Autodesk Inventor part; units mm, degrees
ref_plane "YZ Plane" through (0, 0, 0) normal (1, 0, 0) x (0, 1, 0)
ref_plane "XZ Plane" through (0, 0, 0) normal (0, 1, 0) x (-1, 0, 0)
ref_plane "XY Plane" through (0, 0, 0) normal (0, 0, 1) x (1, 0, 0)
sketch "Sketch1" plane through (0, 0, 0) normal (0, 1, 0) x (-1, 0, 0)
  line L0 (0, 0) -> (88.9, 0)
  line L1 (88.9, 0) -> (76.2, 0) construction
  line L2 (76.2, 0) -> (76.2, -12.7) construction
  line L3 (76.2, -12.7) -> (88.9, -12.7) construction
  line L4 (88.9, -12.7) -> (88.9, 0) construction
  line L5 (0, -349.25) -> (88.9, -349.25) construction
  line L6 (88.9, -698.5) -> (76.2, -698.5) construction
  line L7 (76.2, -698.5) -> (76.2, -685.8) construction
  line L8 (76.2, -685.8) -> (88.9, -685.8) construction
  line L9 (0, 0) -> (12.7, 0) construction
  line L10 (12.7, 0) -> (12.7, -12.7) construction
  line L11 (12.7, -12.7) -> (0, -12.7) construction
  line L12 (0, -12.7) -> (0, 0) construction
  line L13 (0, -698.5) -> (12.7, -698.5) construction
  line L14 (12.7, -698.5) -> (12.7, -685.8) construction
  line L15 (12.7, -685.8) -> (0, -685.8) construction
  line L16 (88.9, -12.7) -> (76.2, -12.7)
  line L17 (76.2, -12.7) -> (76.2, -685.8)
  line L18 (76.2, -685.8) -> (88.9, -685.8)
  line L19 (12.7, -685.8) -> (0, -685.8)
  line L20 (0, -12.7) -> (12.7, -12.7)
  line L21 (12.7, -12.7) -> (12.7, -685.8)
  line L22 (0, -12.7) -> (0, 0)
  line L23 (88.9, 0) -> (88.9, -12.7)
  line L24 (0, -685.8) -> (0, -749.3)
  line L25 (0, -749.3) -> (88.9, -749.3)
  line L26 (88.9, -749.3) -> (88.9, -685.8)
  dimension "d2" = 12.7
  dimension "d3" = 12.7
  dimension "d8" = 88.9
  dimension "d10" = 63.5
extrude "Extrusion1" add sketch "Sketch1" along normal blind 12.7
fillet "Fillet1" radius 6.35 3 edges at (-44.45, 12.7, 0) (-88.9, 12.7, -6.35) (0, 12.7, -6.35)
fillet "Fillet3" radius 6.35 3 edges at (-44.45, 12.7, -749.3) (-88.9, 12.7, -717.55) (0, 12.7, -717.55)
sketch "Sketch2" plane through (0, 12.7, 0) normal (0, 1, 0) x (1, 0, 0)
  line L0 (-88.9, 749.3) -> (0, 749.3) construction
  line L1 (-44.45, 749.2751) -> (-44.45, 698.4751) construction
  line L2 (-44.45, 749.2751) -> (6.35, 749.2751) construction
  line L3 (-44.45, 698.4751) -> (-50.8, 698.4751) construction
  line L4 (-44.45, 698.4751) -> (-38.1, 698.4751) construction
  line L5 (-50.8, 698.4751) -> (-38.1, 698.4751)
  line L6 (-38.1, 698.4751) -> (-38.1, 685.7751)
  line L7 (-38.1, 685.7751) -> (-50.8, 685.7751)
  line L8 (-50.8, 685.7751) -> (-50.8, 698.4751)
  line L9 (-44.45, 685.7751) -> (-44.45, 95.2251) construction
  line L10 (-44.45, 95.2251) -> (-50.8, 95.2251) construction
  line L11 (-44.45, 95.2251) -> (-38.1, 95.2251) construction
  line L12 (-50.8, 95.2251) -> (-38.1, 95.2251)
  line L13 (-38.1, 95.2251) -> (-38.1, 82.5251)
  line L14 (-38.1, 82.5251) -> (-50.8, 82.5251)
  line L15 (-50.8, 82.5251) -> (-50.8, 95.2251)
  line L16 (-44.45, 82.5251) -> (-44.45, 72.6191) construction
  line L17 (-44.45, 82.5251) -> (-34.544, 82.5251) construction
  line L18 (-44.45, 72.6191) -> (-50.8, 72.6191) construction
  line L19 (-44.45, 72.6191) -> (-38.1, 72.6191) construction
  line L20 (-50.8, 72.6191) -> (-38.1, 72.6191)
  line L21 (-38.1, 72.6191) -> (-38.1, 59.9191)
  line L22 (-38.1, 59.9191) -> (-50.8, 59.9191)
  line L23 (-50.8, 59.9191) -> (-50.8, 72.6191)
  line L24 (-44.45, 59.9191) -> (-44.45, 12.6751) construction
  line L25 (-88.9, 0) -> (0, 0) construction
  line L26 (-44.45, 0) -> (-38.1, 0) construction
  line L27 (-44.45, 0) -> (-38.1, 0) construction
  line L28 (-38.1, 0) -> (-50.8, 0)
  line L29 (-50.8, 0) -> (-50.8, 12.7)
  line L30 (-50.8, 12.7) -> (-38.1, 12.7)
  line L31 (-38.1, 12.7) -> (-38.1, 0)
  line L32 (-44.45, 390.5001) -> (67.6838, 390.5001) construction
  dimension "d12" = 50.8
  dimension "d13" = 90
  dimension "d14" = 6.35
  dimension "d15" = 180
  dimension "d16" = 12.7
  dimension "d17" = 12.7
  dimension "d18" = 590.55
  dimension "d20" = 6.35
  dimension "d21" = 180
  dimension "d22" = 12.7
  dimension "d23" = 12.7
  dimension "d24" = 9.906
  dimension "d25" = 90
  dimension "d26" = 6.35
  dimension "d27" = 180
  dimension "d28" = 12.7
  dimension "d29" = 12.7
  dimension "d30" = 6.35
  dimension "d31" = 0
  dimension "d32" = 12.7
  dimension "d33" = 12.7
extrude "Extrusion2" cut sketch "Sketch2" along normal through all both and the other way through all
properties part number "Arm Top" material "PVC-Piping"
Verification items for the finished model (mm, model axes). A direction names the side the tool comes from. Coordinates: 2 decimals unless noted, no trailing zeros. Loops run counter-clockwise (first coordinate to the right, second up) from the corner with the lowest first, then second, coordinate; pieces in that order, holes last. Notation, with made-up numbers: (-29.5, 57.25) -> (29.5, 57.25) arc R23 cw to (29.5, 93.25) -> close; hole circle Ø3 at (34.5, 31). An arc over 180 degrees is marked (long way). Put each result on its own line as item: value.
1. Gauge pin test, flat ends, axial feed: P1, Ø4, axis at x = -45.5, y = 4, coming from the +Z side; P2, Ø1.5, axis at y = 9.5, z = -86.5, coming from the +X side; P3, Ø8, axis at x = -44, z = -374.5, coming from the -Y side; P4, Ø3, axis at y = 9.5, z = -509, coming from the -X side. Record the tip position at first contact, or that the pin passes through.
Result set:
P1: stops at z = -12.7
P2: stops at x = -12.7
P3: stops at y = 0
P4: stops at x = -76.2
2. Section check B-B, the plane z = -551.5. Record the boundary of the cut face in (x, y), then the cut area to 3 significant figures.
Result set:
outline: (-76.2, 0) -> (-12.7, 0) -> (-12.7, 12.7) -> (-76.2, 12.7) -> close
area: 806 mm^2
3. Tool access check on faces 1 (the face through (-83, 6, -12.7)), 2 (the face through (-45, 6, -95.225)), 3 (the face through (-38.1, 6, -6)). Record the directions out of +Z, -Z, +X, -X, +Y, -Y that give a thin tool (end or side, any length) a straight path to the whole face; none if there is none.
Result set:
face 1: -X, +Y, -Y
face 2: +Y, -Y
face 3: +Z, +Y, -Y
4. Section check A-A, the plane y = 3.75. Record the boundary of the cut face in (x, z).
Result set:
outline: (-88.9, -749.3) -> (0, -749.3) -> (0, -685.8) -> (-12.7, -685.8) -> (-12.7, -12.7) -> (0, -12.7) -> (0, 0) -> (-38.1, 0) -> (-38.1, -12.7) -> (-50.8, -12.7) -> (-50.8, 0) -> (-88.9, 0) -> (-88.9, -12.7) -> (-76.2, -12.7) -> (-76.2, -685.8) -> (-88.9, -685.8) -> close; hole (-50.8, -698.48) -> (-38.1, -698.48) -> (-38.1, -685.78) -> (-50.8, -685.78) -> close; hole (-50.8, -95.23) -> (-38.1, -95.23) -> (-38.1, -82.53) -> (-50.8, -82.53) -> close; hole (-50.8, -72.62) -> (-38.1, -72.62) -> (-38.1, -59.92) -> (-50.8, -59.92) -> close
5. Mould release check, pull along Z, two halves, no side actions. Record for faces 4 (the face through (-50.8, 6, -692)), 5 (the face through (-44, 12.7, -369)), 6 (the face through (-45, 6, -12.7)): pulls with the +Z half, pulls with the -Z half, needs draft (parallel to the pull), parting line crosses it, or undercut.
Result set:
face 4: undercut
face 5: needs draft
face 6: pulls with the +Z half
6. Thickness scan on line 1 (Z direction, x = -83, y = 4.5); line 2 (Z direction, x = -41.5, y = 7.25); line 3 (Z direction, x = -50, y = 10.5). Record the ranges inside material, lowest first.
Result set:
line 1: z = -749.3 to -685.8, -12.7 to 0
line 2: z = -749.24 to -698.48, -685.78 to -95.23, -82.53 to -72.62, -59.92 to -12.7
line 3: z = -747.76 to -698.48, -685.78 to -95.23, -82.53 to -72.62, -59.92 to -12.7
